Work out the finished part from the listing and answer in its coordinate system (mm). A direction names the side the tool comes from. Coordinates: 2 decimals unless noted, no trailing zeros. Write each loop counter-clockwise with the first axis right and the second up, starting at its lowest first coordinate (ties: lowest second). Pieces come first, ordered by that corner, then holes. Notation, with made-up numbers: (55.25, -34.5) - (81.25, -34.5) arc R12 ccw to (81.25, -19.5) - close; hole circle Ø4 at (24.25, -8). An arc over 180 degrees is marked (long way). Answer as a JSON object with one key per item and string values. Group by question number.
from build123d import *

# Parameters (mm, degrees)
ESQUISSE1_W             = 10
ESQUISSE1_H             = 80
BOSS_EXTRU_1_DEPTH      = 10
BOSS_EXTRU_2_DEPTH      = 10
CONG_1_R                = 26.656312
ESQUISSE4_R             = 1.5
ENL_V_MAT_EXTRU_2_DEPTH = 118.473401245
ESQUISSE7_R             = 1.025
BOSS_EXTRU_3_DEPTH      = 10
CONG_2_R                = 3
CONG_3_R                = 3
CONG_4_R                = 5
CONG_5_R                = 57
CONG_6_R                = 57


with BuildPart() as part:
    # Esquisse1 → Boss.-Extru.1 (new body)
    with BuildSketch(Plane.XY):
        Rectangle(ESQUISSE1_W, ESQUISSE1_H)
    extrude(amount=BOSS_EXTRU_1_DEPTH)

    # Esquisse2 → Boss.-Extru.2 (add, through all)
    with BuildSketch(Plane.ZY.offset(5)):
        Polygon((10, 40), (110, 22.367301929), (110, -22.367301929), (10, -40), align=None)
        with BuildLine():
            Line((25, 25), (25, -25))
            ThreePointArc((25, -25), (20, -30), (15, -25))
            Line((15, -25), (15, 25))
            ThreePointArc((15, 25), (20, 30), (25, 25))
        make_face(mode=Mode.SUBTRACT)
        with BuildLine():
            Line((45, 15), (85, 15))
            ThreePointArc((85, 15), (92.071067812, 12.071067812), (95, 5))
            Line((95, 5), (95, -5))
            ThreePointArc((95, -5), (92.071067812, -12.071067812), (85, -15))
            Line((85, -15), (45, -15))
            ThreePointArc((45, -15), (37.928932188, -12.071067812), (35, -5))
            Line((35, -5), (35, 5))
            ThreePointArc((35, 5), (37.928932188, 12.071067812), (45, 15))
        make_face(mode=Mode.SUBTRACT)
    extrude(amount=-BOSS_EXTRU_2_DEPTH)

    # Congé1
    cong_1_edges = [part.edges().sort_by_distance(p)[0] for p in [
        (0, 22.367301929, 110),
        (0, -22.367301929, 110),
    ]]
    fillet(cong_1_edges, radius=CONG_1_R)

    # Esquisse4 → Enlèv. mat.-Extru.2 (cut, through all)
    with BuildSketch(Plane(origin=(5, 0, 0), x_dir=(0, 0, -1), z_dir=(1, 0, 0))):
        with Locations(Location((-5, -26.578661355, 0), (0, 0, 90))):
            Circle(ESQUISSE4_R)
    extrude(amount=-ENL_V_MAT_EXTRU_2_DEPTH, mode=Mode.SUBTRACT)

    # Esquisse7 → Boss.-Extru.3 (add, through all)
    with BuildSketch(Plane(origin=(5, 0, 0), x_dir=(0, 0, -1), z_dir=(1, 0, 0))):
        with BuildLine():
            Line((3.625, 28.948557159), (0, 31.041451884))
            Line((0, 31.041451884), (0, 22.958548116))
            Line((0, 22.958548116), (3.625, 25.051442841))
            ThreePointArc((3.625, 25.051442841), (4.75, 27), (3.625, 28.948557159))
        make_face()
        with Locations(Location((2.5, 27, 0), (0, 0, 90))):
            Circle(ESQUISSE7_R, mode=Mode.SUBTRACT)
    extrude(amount=-BOSS_EXTRU_3_DEPTH)

    # Congé2
    cong_2_edges = [part.edges().sort_by_distance(p)[0] for p in [
        (0, 22.958548116, 0),
    ]]
    fillet(cong_2_edges, radius=CONG_2_R)

    # Congé3
    cong_3_edges = [part.edges().sort_by_distance(p)[0] for p in [
        (0, 31.041451884, 0),
    ]]
    fillet(cong_3_edges, radius=CONG_3_R)

    # Congé4
    cong_4_edges = [part.edges().sort_by_distance(p)[0] for p in [
        (0, -40, 0),
        (0, 40, 0),
    ]]
    fillet(cong_4_edges, radius=CONG_4_R)

    # Congé5
    cong_5_edges = [part.edges().sort_by_distance(p)[0] for p in [
        (0, 40, 10),
    ]]
    fillet(cong_5_edges, radius=CONG_5_R)

    # Congé6
    cong_6_edges = [part.edges().sort_by_distance(p)[0] for p in [
        (0, -40, 10),
    ]]
    fillet(cong_6_edges, radius=CONG_6_R)


solid = part.part
Q1. Section C-C on y = -17 is taken. Determine the outline of the cut face in (x, z).
Q2. A tool of negligible diameter and unlimited length cuts with its end or side. For faces 5 (the face through (0, 0, 25)), 6 (the face through (0, -6, 0)), 7 (the face through (5, 1, 28)), from which of +Z, -Z, +X, -X, +Y, -Y can it reach the whole face along a straight path? Write none if from no direction.
Q3. Section B-B on z = 20 is taken. Determine the outline of the cut face in (x, y), plus the area to 3 significant figures.
Q4. Flat-ended cylindrical pins translate along their axes: pin 1 Ø6 at (y, z) = (-5, 37) entering from -X; pin 2 Ø2 at (x, z) = (0.5, 72.5) entering from +Y; pin 3 Ø3 at (x, y) = (-1, -8) entering from -Z; pin 4 Ø3 at (x, z) = (-2, 58) entering from -Y. Find the tip coordinate at first contact, or state that the pin passes through.
Q5. For a pull along Z with two mould halves and no side action, classify faces 1 (the face through (-5, 1, 28)), 2 (the face through (0, -15, 65)), 3 (the face through (0.07, 39.79, 9.91)), 4 (the face through (0, 0, 15)) as +Z half, -Z half, draft (parallel to the pull), parting line (faces both ways), or undercut.
Q6. Section A-A on x = -0.75 is taken. Count the separate pieces of the cut face and the enclosed holes in it, plus the area to 3 significant figures.
Q7. Consider L1, parallel to Z at x = -2, y = 5.5; L2, parallel to Y at x = -1, z = 82; L3, parallel to Z at x = -2, y = -5. Determine where each line is inside the solid, lowest interval first. Write a range as from..to.
Numbers:
{
 "1": {"outline": "(-5, 0) - (5, 0) - (5, 15) - (-5, 15) - close; (-5, 25) - (5, 25) - (5, 103.88) - (-5, 103.88) - close"},
 "2": {"face 5": "+X, -X", "face 6": "-Z, +X, -X, -Y", "face 7": "+Z, -Z, +X, +Y, -Y"},
 "3": {"outline": "(-5, -38.24) - (5, -38.24) - (5, -30) - (-5, -30) - close; (-5, 30) - (5, 30) - (5, 38.24) - (-5, 38.24) - close", "area": "165 mm²"},
 "4": {"pin 1": "stops at x = -5", "pin 2": "stops at y = 29.16", "pin 3": "stops at z = 0", "pin 4": "stops at y = -31.8"},
 "5": {"face 1": "draft", "face 2": "undercut", "face 3": "+Z half", "face 4": "undercut"},
 "6": {"separate pieces": "1", "enclosed holes": "4", "area": "4,550 mm²"},
 "7": {"L1": "z = 0..15, 25..35.01, 94.99..109.43", "L2": "y = -27.3..-15, 15..27.3", "L3": "z = 0..15, 25..35, 95..109.53"}
}
